```python
from build123d import *

# Parameters (mm, degrees)
F0_W     = 10
F0_H     = 18
F1_DEPTH = 4
F3_DEPTH = 18.001
F4_W     = 10
F4_H     = 6
F5_DEPTH = 2


with BuildPart() as f1:
    # F0 (on Top) → F1 (new body)
    with BuildSketch(Plane.XY):
        Rectangle(F0_W, F0_H)
    extrude(amount=F1_DEPTH)

    # F2 (on face) → F3 (intersect, through all)
    with BuildSketch(Plane.XZ.offset(9)):
        Polygon((5, 2), (-5, 0.5), (-5, 0), (5, 0), align=None)
    extrude(amount=-F3_DEPTH, mode=Mode.INTERSECT)

    # F4 (on face) → F5 (join)
    with BuildSketch(Plane(origin=(0, 0, 0), x_dir=(1, 0, 0), z_dir=(0, 0, -1))):
        Rectangle(F4_W, F4_H)
    extrude(amount=F5_DEPTH)


solid = f1.part
```
CAD build for the part. Positions are in the model's coordinates, mm. A direction names the side the tool comes from. Round coordinates to 2 decimals unless told otherwise and drop trailing zeros. Loops run counter-clockwise (first coordinate to the right, second up) from the corner with the lowest first, then second, coordinate; pieces in that order, holes last. Notation, with made-up numbers: M 35.5,11.25 L 87.5,11.25 A9 cw 87.5,25.25 Z; hole C 35,-36.5 d8. An arc over 180 degrees is marked long. Return JSON: item names as keys, results as strings. Group by question number.
(1) Drop flat-ended pins along their axis: P1, Ø2, axis at x = -2.5, z = -1.5, coming from the +Y side; P2, Ø1.8, axis at x = -1.5, y = -5, coming from the -Z side; P3, Ø5, axis at x = -2.5, y = -4, coming from the +Z side. Give the stop position or say it passes through.
(2) Saw through at B-B, the plane z = 0.8. List the corners of the cut face in (x, y), and give its area (3 significant figures).
(3) Saw through at D-D, the plane x = 1.5. List the corners of the cut face in (y, z) (3 decimals).
(4) Saw through at C-C, the plane y = -6. List the corners of the cut face in (x, z).
(5) Wall check: probe 1 along Y at (x, z) = (-1.5, -1); probe 2 along Z at (x, y) = (-2.75, 5.5); probe 3 along Z at (x, y) = (0.75, 5). Give the ranges that are in metal, low to high. Write a range as [from, to].
(6) Saw through at A-A, the plane x = -1. List the corners of the cut face in (y, z), and give its area (3 significant figures).
(7) Tool access for faces 1 (the flat face through (0, 6, 0)), 2 (the flat face through (5, 0, 0)), 3 (the flat face through (0, -3, -1)): list every direction of +Z, -Z, +X, -X, +Y, -Y with a clear straight run to the whole face (end or side of a thin tool).
Answer list:
{
 "1": {"P1": "y = 3", "P2": "z = 0", "P3": "z = 1.25"},
 "2": {"outline": "M -3,-9 L 5,-9 L 5,9 L -3,9 Z", "area": "144 mm2"},
 "3": {"outline": "M -9,0 L -3,0 L -3,-2 L 3,-2 L 3,0 L 9,0 L 9,1.475 L -9,1.475 Z"},
 "4": {"outline": "M -5,0 L 5,0 L 5,2 L -5,0.5 Z"},
 "5": {"probe 1": "[-3, 3]", "probe 2": "[0, 0.84]", "probe 3": "[0, 1.36]"},
 "6": {"outline": "M -9,0 L -3,0 L -3,-2 L 3,-2 L 3,0 L 9,0 L 9,1.1 L -9,1.1 Z", "area": "31.8 mm2"},
 "7": {"face 1": "-Z, +X, -X, +Y", "face 2": "+Z, -Z, +X, +Y, -Y", "face 3": "-Z, +X, -X, -Y"}
}
